Solid Edge part; units mm, degrees
sketch "Sketch1" plane through (0, 0, 0) normal (0, -1, 0) x (1, 0, 0)
  line L0 (-36, 0) -> (0, 0)
  line L1 (0, 0) -> (0, 36)
  line L2 (0, 36) -> (4, 36)
  line L3 (4, 36) -> (4, -4)
  line L4 (4, -4) -> (-36, -4)
  line L5 (-36, -4) -> (-36, 0)
extrude "Protrusion1" add sketch "Sketch1" along normal mid plane 350
sketch "Sketch2" plane through (-18, 0, 0) normal (0, 0, 1) x (0, -1, 0)
  circle A0 centre (-155, 2) radius 4
  dimension "D1" = 155
  dimension "D2" = 155
extrude "Cutout1" cut sketch "Sketch2" against normal through all
mirror "Mirror1" about plane through (0, 0, 0) normal (0, -1, 0) of "Cutout1"
sketch "Sketch3" plane through (0, 0, 18) normal (-1, 0, 0) x (0, -1, 0)
  line L0 (-22.5, -18) -> (22.5, -18)
  line L1 (22.5, -18) -> (22.5, 18)
  line L2 (22.5, 18) -> (-22.5, 18)
  line L3 (-22.5, 18) -> (-22.5, -18)
  dimension "D1" = 22.5
extrude "Cutout2" cut sketch "Sketch3" against normal through all
chamfer "Chamfer1" distance 2 angle 45 2 edges at (-18, -175, 0) (-18, 175, 0)
chamfer "Fase_2" distance 2 angle 45 2 edges at (0, -175, 17) (0, 175, 17)
sketch "Sketch4" plane through (0, -97.75, 18) normal (-1, 0, 0) x (0, -1, 0)
  circle A0 centre (-58.75, 5) radius 2.5
  circle A1 centre (-58.75, -10) radius 2.5
  dimension "D1" = 58.75
extrude "Cutout3" cut sketch "Sketch4" against normal through all
properties material "Aluminium, 7075-T6"
Model file for the job. Use its own axes, mm. A direction names the side the tool comes from. Give positions to 0.01 mm unless a question says otherwise; leave off trailing zeros. Order: outer loops, then holes, each group sorted by start corner. A loop starts at its lowest first (then second) coordinate and runs counter-clockwise, first axis right, second up. Notation, with made-up numbers: M -23.5,0.25 L 28.5,0.25 A30 ccw 28.5,25.25 Z; hole C 75.5,49 d7. An arc over 180 degrees is marked long. Put each result on its own line as item: value. Start each with the question number.
(1) Tool access for faces 5 (the face through (-16, 2, -4)), 6 (the face through (0, -97, 18)): list every direction of +Z, -Z, +X, -X, +Y, -Y with a clear straight run to the whole face (end or side of a thin tool).
(2) Pin check, flat tips, straight feed: pin 1 Ø6.5 at (x, y) = (-16, 155) entering from -Z; pin 2 Ø11 at (y, z) = (-125, 21.5) entering from -X; pin 3 Ø5 at (x, y) = (-10.5, 136) entering from +Z. Stop position of each tip, or through.
(3) Band-saw the part on B-B on y = 155. Give the cut face in (x, z), then the cut area to 3 significant figures.
(4) Drill centre lines: L1, parallel to Z at x = 3, y = -39; L2, parallel to Y at x = 2.5, z = 23.5; L3, parallel to X at y = -155, z = -2.1. Where is each one in solid material? Low to high. Write a range as [from, to].
(5) Pull direction X, two halves, no side cores. Call faces 1 (the face through (4, 2, -1)), 2 (the face through (-17.201, -151.185, -1.972)), 3 (the face through (0, 99, 18)), 4 (the face through (-14.799, 151.185, -1.972)): released by +X, released by -X, zero draft, split by the parting line, or undercut.
(6) Band-saw the part on A-A on z = 17. Give the cut face in (x, y).
(7) Band-saw the part on C-C on x = -28. Give the cut face in (y, z), then the cut area to 3 significant figures.
(8) Band-saw the part on D-D on y = -142. Give the cut face in (x, z).
Results below:
1. face 5: -Z, +X, -X, +Y, -Y
1. face 6: +Z, -X, +Y, -Y
2. pin 1: passes through
2. pin 2: stops at x = 0
2. pin 3: stops at z = 0
3. outline: M -36,-4 L -20,-4 L -20,0 L -36,0 Z; M -12,-4 L 4,-4 L 4,36 L 0,36 L 0,0 L -12,0 Z
3. area: 272 mm2
4. L1: z = [-4, 5.5], [10.5, 20.5], [25.5, 36]
4. L2: y = [-175, -41.45], [-36.55, -22.5], [22.5, 175]
4. L3: x = [-36, -20], [-12, 4]
5. face 1: released by +X
5. face 2: undercut
5. face 3: released by -X
5. face 4: undercut
6. outline: M 0,-173 L 2,-175 L 4,-175 L 4,-22.5 L 0,-22.5 Z; M 0,22.5 L 4,22.5 L 4,175 L 2,175 L 0,173 Z
7. outline: M -175,-4 L 175,-4 L 175,-2 L 173,0 L -173,0 L -175,-2 Z
7. area: 1,400 mm2
8. outline: M -36,-4 L 4,-4 L 4,36 L 0,36 L 0,0 L -36,0 Z
